```python
from build123d import *

# Parameters (mm, degrees)
SKETCH2_R           = 50
BOSS_EXTRUDE1_DEPTH = 10
SKETCH4_W           = 30
SKETCH4_H           = 30
CUT_EXTRUDE4_DEPTH  = 72.414284285
SKETCH4_5_W         = 15
SKETCH4_5_H         = 30
SKETCH4_5_W_2       = 30
SKETCH4_5_H_2       = 15
CUT_EXTRUDE5_DEPTH  = 5


with BuildPart() as part:
    # Sketch2 → Boss-Extrude1 (new body)
    with BuildSketch(Plane(origin=(0, 0, 0), x_dir=(1, 0, 0), z_dir=(0, 1, 0))):
        with Locations(Location((0, 0, 0), (0, 0, 270))):
            Circle(SKETCH2_R)
    extrude(amount=BOSS_EXTRUDE1_DEPTH)

    # Sketch4 → Cut-Extrude4 (cut, through all)
    with BuildSketch(Plane.XZ):
        Rectangle(SKETCH4_W, SKETCH4_H)
    extrude(amount=-CUT_EXTRUDE4_DEPTH, mode=Mode.SUBTRACT)

    # Sketch4_5 → Cut-Extrude5 (cut)
    with BuildSketch(Plane.XZ):
        with Locations((-22.5, 0)):
            Rectangle(SKETCH4_5_W, SKETCH4_5_H)
        with Locations((0, -22.5)):
            Rectangle(SKETCH4_5_W_2, SKETCH4_5_H_2)
        with Locations((22.5, 0)):
            Rectangle(SKETCH4_5_W, SKETCH4_5_H)
        with Locations((0, 22.5)):
            Rectangle(SKETCH4_5_W_2, SKETCH4_5_H_2)
    extrude(amount=-CUT_EXTRUDE5_DEPTH, mode=Mode.SUBTRACT)


solid = part.part
```
The model under review builds one solid part; all positions refer to its coordinate system, in mm. A direction names the side the tool comes from. Coordinates: 2 decimals unless noted, no trailing zeros. Write each loop counter-clockwise with the first axis right and the second up, starting at its lowest first coordinate (ties: lowest second). Pieces come first, ordered by that corner, then holes.
1) Machinability: for faces 4 (the face through (0, 7, -15)), 5 (the face through (15, 2, 22)), which of the approach directions +Z, -Z, +X, -X, +Y, -Y give a long, thin tool a straight path to every point of the face, cutting with its end or side? Answer none if there is none.
2) To check wall thickness, follow probe 1 along Y at (x, z) = (-27.5, -5); probe 2 along X at (y, z) = (8.25, 0); probe 3 along Z at (x, y) = (-1, 6.5). State the ranges of each line that lie inside material, in increasing order.
3) We need section D-D on x = -17.5. State the section outline as (y, z) points.
4) Clearance check with flat-ended pins moving along their axes: pin 1 Ø4 at (y, z) = (2.5, 21) entering from -X; pin 2 Ø1 at (x, y) = (7.5, 7) entering from -Z; pin 3 Ø5.5 at (x, y) = (24.5, 2.5) entering from +Z. State where each tip first meets the part, or that it passes through.
5) We need section C-C on y = 2.75. State the section outline as (x, z) points, then the cut area to 3 significant figures.
6) We need section B-B on x = 0. State the section outline as (y, z) points.
7) The part is to be moulded in two halves that separate along Z. For faces 1 (the face through (-22, 0, 22)), 2 (the face through (15.02, 4.93, 47.69)), 3 (the face through (-23, 5, 0)), say which applies: pulls with the +Z half, pulls with the -Z half, needs draft (parallel to the pull), parting line crosses it, or undercut.
8) We need section A-A on z = 0. State the section outline as (x, y) points.
Answer list:
1. face 4: +Y, -Y
1. face 5: -Y
2. probe 1: y = 5 to 10
2. probe 2: x = -50 to -15, 15 to 50
2. probe 3: z = -49.99 to -15, 15 to 49.99
3. outline: (0, -46.84) - (10, -46.84) - (10, 46.84) - (0, 46.84) - (0, 15) - (5, 15) - (5, -15) - (0, -15) - close
4. pin 1: stops at x = -46.25
4. pin 2: stops at z = -49.51
4. pin 3: stops at z = 45.02
5. outline: circle Ø100 at (0, 0); hole (-30, -15) - (-15, -15) - (-15, -30) - (15, -30) - (15, -15) - (30, -15) - (30, 15) - (15, 15) - (15, 30) - (-15, 30) - (-15, 15) - (-30, 15) - close
5. area: 5,150 mm2
6. outline: (0, -50) - (10, -50) - (10, -15) - (5, -15) - (5, -30) - (0, -30) - close; (0, 30) - (5, 30) - (5, 15) - (10, 15) - (10, 50) - (0, 50) - close
7. face 1: needs draft
7. face 2: parting line crosses it
7. face 3: undercut
8. outline: (-50, 0) - (-30, 0) - (-30, 5) - (-15, 5) - (-15, 10) - (-50, 10) - close; (15, 5) - (30, 5) - (30, 0) - (50, 0) - (50, 10) - (15, 10) - close
